```python
from build123d import *

# Parameters (mm, degrees)
F0_W     = 152.4
F0_H     = 190.5
F1_DEPTH = 5.08
F2_W     = 38.1
F2_H     = 38.1
F2_R     = 19.05
F2_W_2   = 25.4
F3_DEPTH = 25.4


with BuildPart() as f1:
    # F0 (on Top) → F1 (new body)
    with BuildSketch(Plane.XY):
        with Locations((-10.361006, 12.33527)):
            Rectangle(F0_W, F0_H)
    extrude(amount=F1_DEPTH)

    # F2 (on face) → F3 (cut)
    with BuildSketch(Plane.XY.offset(5.08)):
        with Locations((23.089969, 61.145121)):
            Rectangle(F2_W, F2_H)
        Polygon((19.348822, -67.770637), (0.298822, -34.775069), (-18.751178, -67.770637), align=None)
        with Locations((-37.642254, 59.088646)):
            Circle(F2_R)
        Polygon((15.868925, -21.180481), (37.180649, -15.732507), (43.118428, 5.447974), (27.744482, 21.180481), (6.432758, 15.732507), (0.49498, -5.447974), align=None)
        with Locations((-46.103996, -9.714661)):
            Rectangle(F2_W_2, F2_H)
    extrude(amount=-F3_DEPTH, mode=Mode.SUBTRACT)


solid = f1.part
```
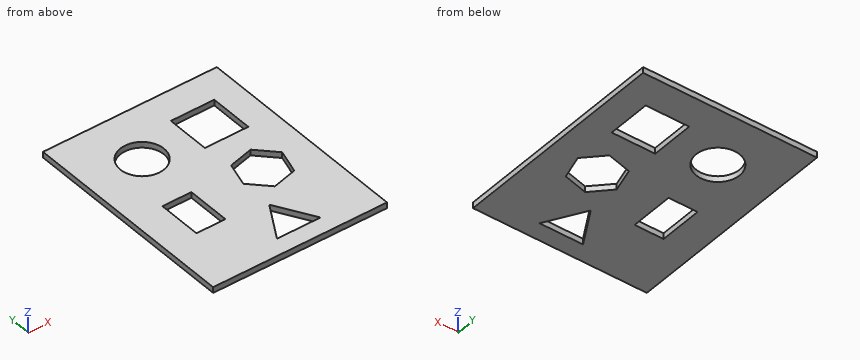
Source: CAD feature listing. Evaluate the final solid. Frame: model axes, mm. Give positions to 0.01 mm unless a question says otherwise; leave off trailing zeros. Loops run counter-clockwise (first coordinate to the right, second up) from the corner with the lowest first, then second, coordinate; pieces in that order, holes last. Notation, with made-up numbers: (81.5, 44.5) -> (125.5, 44.5) arc R17 cw to (125.5, 60.5) -> close; hole circle Ø6 at (-8, -6.75). An arc over 180 degrees is marked (long way). Use a Markdown table: item, result. Add a question column.
(1) Ray query, line 1 (X direction, y = 58.5, z = 3.25); line 2 (X direction, y = -27, z = 0.65); line 3 (Y direction, x = -35.5, z = 0.85). Return the intervals inside material, ascending.
(2) Section query A-A (y = -44). Output: boundary loops of the cut face in (x, z), then the cut area to 3 significant figures.
(3) Section query C-C (y = 49). Output: boundary loops of the cut face in (x, z).
(4) Section query B-B (x = -52). Output: boundary loops of the cut face in (y, z).
(5) Section query D-D (x = -27). Output: boundary loops of the cut face in (y, z), then the cut area to 3 significant figures.
Checked values:
| question | item | result |
|---|---|---|
| 1 | line 1 | -86.56 to -56.68, -18.6 to 4.04, 42.14 to 65.84 |
| 1 | line 2 | -86.56 to -58.8, -33.4 to 65.84 |
| 1 | line 3 | -82.91 to -28.76, 9.34 to 40.16, 78.02 to 107.59 |
| 2 | outline | (-86.56, 0) -> (-5.03, 0) -> (-5.03, 5.08) -> (-86.56, 5.08) -> close; (5.62, 0) -> (65.84, 0) -> (65.84, 5.08) -> (5.62, 5.08) -> close |
| 2 | area | 720 mm^2 |
| 3 | outline | (-86.56, 0) -> (-53.8, 0) -> (-53.8, 5.08) -> (-86.56, 5.08) -> close; (-21.48, 0) -> (4.04, 0) -> (4.04, 5.08) -> (-21.48, 5.08) -> close; (42.14, 0) -> (65.84, 0) -> (65.84, 5.08) -> (42.14, 5.08) -> close |
| 4 | outline | (-82.91, 0) -> (-28.76, 0) -> (-28.76, 5.08) -> (-82.91, 5.08) -> close; (9.34, 0) -> (46.57, 0) -> (46.57, 5.08) -> (9.34, 5.08) -> close; (71.61, 0) -> (107.59, 0) -> (107.59, 5.08) -> (71.61, 5.08) -> close |
| 5 | outline | (-82.91, 0) -> (43.29, 0) -> (43.29, 5.08) -> (-82.91, 5.08) -> close; (74.89, 0) -> (107.59, 0) -> (107.59, 5.08) -> (74.89, 5.08) -> close |
| 5 | area | 807 mm^2 |
